The drawing under review shows one solid part. Ordinate dimensions are in mm from its lowest x, y, z. Round coordinates to 2 decimals unless told otherwise and drop trailing zeros. Order: outer loops, then holes, each group sorted by start corner. A loop starts at its lowest first (then second) coordinate and runs counter-clockwise, first axis right, second up. Notation, with made-up numbers: (37.25, 0.25) -> (80.25, 0.25) arc R19 ccw to (80.25, 33.25) -> close; hole circle Ø8 at (68.5, 14). An arc over 180 degrees is marked (long way). Return JSON: item names as keys, results as strings. Group by question number.
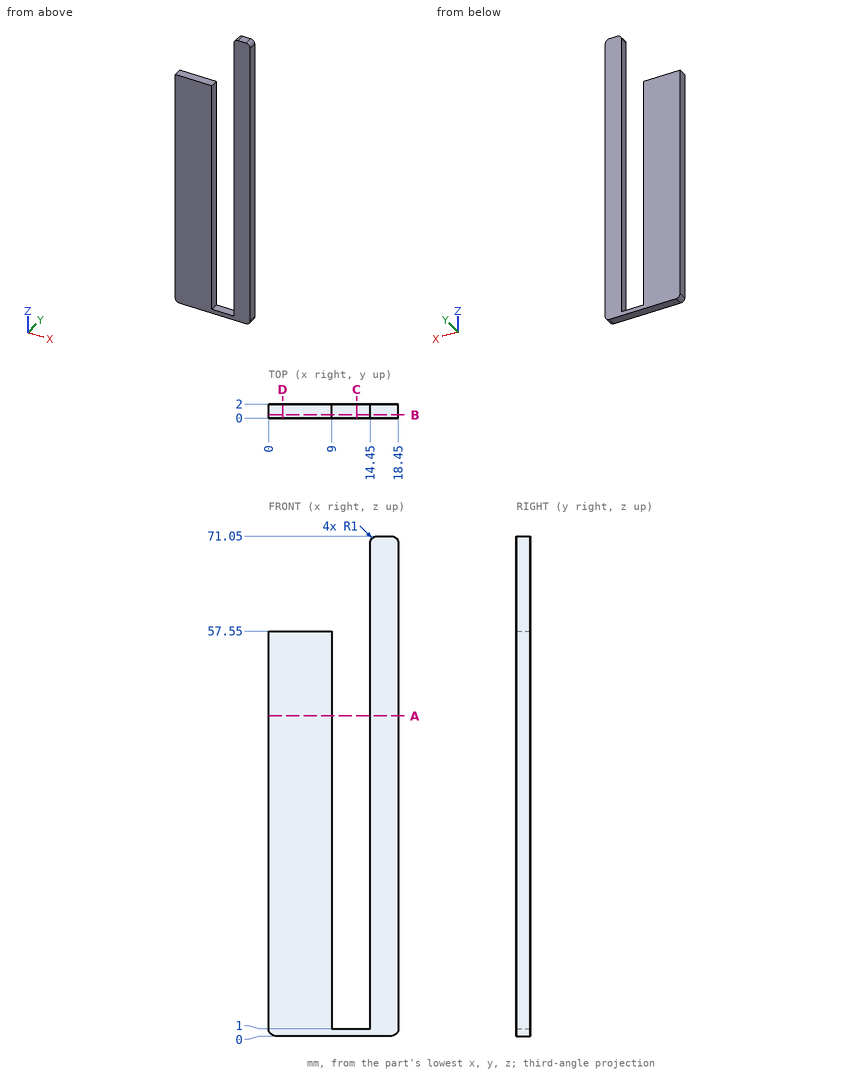
Item 1: Insertion check: pin 1 Ø4 at (x, z) = (11.5, 19.5) entering from +Y; pin 2 Ø0.6 at (x, y) = (11.5, 1.5) entering from +Z; pin 3 Ø0.6 at (x, y) = (3.5, 0.5) entering from +Z. Each pin has a flat end and moves straight along its axis. Give the tip position at first contact, or say it passes through.
Item 2: Consider section C-C on x = 12.5. State the section outline as (y, z) points.
Item 3: Wall thickness on line 1 along X through (y, z) = (1.95, 22); line 2 along Z through (x, y) = (11.5, 1.05); line 3 along Z through (x, y) = (4.75, 0.75): over which ranges is each line inside the solid? List them lowest first.
Item 4: Consider section A-A on z = 45.5. State the section outline as (x, y) points.
Item 5: Consider section B-B on y = 0.45. State the section outline as (x, z) points.
Item 6: Consider section D-D on x = 2. State the section outline as (y, z) points.
Values:
{
 "1": {"pin 1": "through", "pin 2": "z = 1", "pin 3": "z = 57.55"},
 "2": {"outline": "(0, 0) -> (2, 0) -> (2, 1) -> (0, 1) -> close"},
 "3": {"line 1": "0 to 9, 14.45 to 18.45", "line 2": "0 to 1", "line 3": "0 to 57.55"},
 "4": {"outline": "(0, 0) -> (9, 0) -> (9, 2) -> (0, 2) -> close; (14.45, 0) -> (18.45, 0) -> (18.45, 2) -> (14.45, 2) -> close"},
 "5": {"outline": "(0, 1) arc R1 ccw to (1, 0) -> (17.45, 0) arc R1 ccw to (18.45, 1) -> (18.45, 70.05) arc R1 ccw to (17.45, 71.05) -> (15.45, 71.05) arc R1 ccw to (14.45, 70.05) -> (14.45, 1) -> (9, 1) -> (9, 57.55) -> (0, 57.55) -> close"},
 "6": {"outline": "(0, 0) -> (2, 0) -> (2, 57.55) -> (0, 57.55) -> close"}
}
